from build123d import *

# Parameters (mm, degrees)
F9_R      = 2.740867
F10_DEPTH = 75
F11_DEPTH = 2.5


with BuildPart() as f3:
    # F2 (on offset) → F3 section 0
    with BuildSketch(Plane.XY.offset(-50)):
        with BuildLine():
            ThreePointArc((30.178057, -85.267261), (22.527556, -33.46393), (0, 13.807885))
            ThreePointArc((0, 13.807885), (-22.527556, -33.46393), (-30.178057, -85.267261))
            Line((-30.178057, -85.267261), (-25.33818, -85.267261))
            ThreePointArc((-25.33818, -85.267261), (-17.332774, -41.247761), (0, 0))
            ThreePointArc((0, 0), (17.332774, -41.247761), (25.33818, -85.267261))
            Line((25.33818, -85.267261), (30.178057, -85.267261))
        make_face()
    # F0 (on Top) → F3 section 1
    with BuildSketch(Plane.XY):
        with BuildLine():
            Line((11.943851, -95.035806), (37.024528, -95.035806))
            ThreePointArc((37.024528, -95.035806), (28.659989, -20.101697), (0, 49.638472))
            ThreePointArc((0, 49.638472), (-28.659989, -20.101697), (-37.024528, -95.035806))
            Line((-37.024528, -95.035806), (-11.943851, -95.035806))
            Line((-11.943851, -95.035806), (0, -32.345828))
            Line((0, -32.345828), (11.943851, -95.035806))
        make_face()
    loft()

    # F6 (on offset) → F7 section 0
    with BuildSketch(Plane.XY.offset(-40)):
        with BuildLine():
            ThreePointArc((28.793208, -83.320476), (21.105687, -34.645532), (0, 9.884212))
            ThreePointArc((0, 9.884212), (-21.105687, -34.645532), (-28.793208, -83.320476))
            Line((-28.793208, -83.320476), (-25.807247, -82.68062))
            ThreePointArc((-25.807247, -82.68062), (-18.222281, -39.094475), (0, 1.219694))
            ThreePointArc((0, 1.219694), (18.222281, -39.094475), (25.807247, -82.68062))
            Line((25.807247, -82.68062), (28.793208, -83.320476))
        make_face()
    # F4 (on Top) → F7 section 1
    with BuildSketch(Plane.XY):
        with BuildLine():
            Line((15.356379, -90.572096), (33.698723, -90.572096))
            ThreePointArc((33.698723, -90.572096), (24.74767, -22.13133), (0, 42.303231))
            ThreePointArc((0, 42.303231), (-24.74767, -22.13133), (-33.698723, -90.572096))
            Line((-33.698723, -90.572096), (-15.356379, -90.572096))
            Line((-15.356379, -90.572096), (0, -24.667639))
            Line((0, -24.667639), (15.356379, -90.572096))
        make_face()
    loft(mode=Mode.SUBTRACT)

    # F9 (on offset) → F10 (join)
    with BuildSketch(Plane.XY.offset(-25)):
        with Locations((0, -11.576544)):
            Circle(F9_R)
    extrude(amount=F10_DEPTH)

    # F9 (on offset) → F11 (join)
    with BuildSketch(Plane.XY.offset(-25)):
        with Locations((0, -11.576544)):
            Circle(F9_R)
    extrude(amount=-F11_DEPTH)


solid = f3.part
The model under review builds one solid part; all positions refer to its coordinate system, in mm. Coordinates: 2 decimals unless noted, no trailing zeros. Loops run counter-clockwise (first coordinate to the right, second up) from the corner with the lowest first, then second, coordinate; pieces in that order, holes last. Notation, with made-up numbers: M -18.75,13 L 2.25,13 A9 cw 2.25,24 Z; hole C 74.5,1.5 d1. An arc over 180 degrees is marked long. Put each result on its own line as item: value. Start each with the question number.
Q1. Wall thickness on line 1 (X direction, y = -49.5, z = -32); line 2 (X direction, y = -17, z = -13); line 3 (X direction, y = -77.5, z = -36): over which ranges is each line inside the solid? List them lowest first.
Q2. Add section A-A (z = -4.5). Count the separate pieces of the cut face and the enclosed holes in it, and give its area (3 significant figures).
Q3. Clearance check with flat-ended pins moving along their axes: pin 1 (3 mm diameter, centred on x = -23.5, y = -7, fed in from +Z); pin 2 (5 mm diameter, centred on y = 11.5, z = -33.5, fed in from -X); pin 3 (2 mm diameter, centred on y = -34.5, z = -4.5, fed in from -X). State where each tip first meets the part, or that it passes through.
Q4. Add section B-B (z = 24.5). Write out the cut boundary in (x, y), and give its area (3 significant figures).
Q5. The part is to be moulded in two halves that separate along X. For faces 1 (the flat face through (-1, -34, 0)), 2 (the flat face through (-16, -30, -40)), say which applies: +X half, -X half, draft (parallel to the pull), parting line (faces both ways), or undercut.
Answers:
1. line 1: x = -29.5 to -26.09, -17.97 to -13.29, 13.29 to 17.97, 26.09 to 29.5
1. line 2: x = -25.22 to -20.91, -0.27 to 0.27, 20.91 to 25.22
1. line 3: x = -31.95 to -29.08, -24.3 to -20.34, 20.34 to 24.3, 29.08 to 31.95
2. separate pieces: 2
2. enclosed holes: 1
2. area: 1,750 mm^2
3. pin 1: stops at z = 0
3. pin 2: stops at x = -9.8
3. pin 3: stops at x = -31.43
4. outline: C 0,-11.58 d5.48
4. area: 23.6 mm^2
5. face 1: draft
5. face 2: undercut
